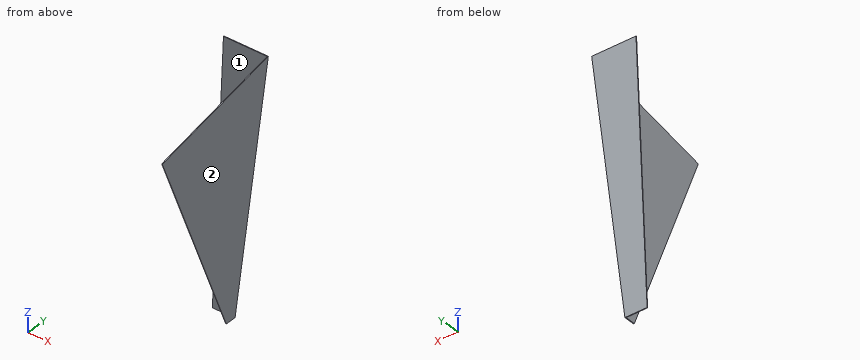
```python
from build123d import *

# Parameters (mm, degrees)
F1_DEPTH = 3.175
F3_DEPTH = 609.6
F5_DEPTH = 1211.58
F7_DEPTH = 25.4


with BuildPart() as f1:
    # F0 (on Front) → F1 (new body)
    with BuildSketch(Plane.XZ):
        Polygon((50.8, -609.6), (203.2, 609.6), (0, 609.6), (0, -609.6), align=None)
        Polygon((0, -609.6), (0, 609.6), (-203.2, 609.6), (-50.8, -609.6), align=None)
    extrude(amount=F1_DEPTH)

    # F2 (on face) → F3 (join)
    with BuildSketch(Plane.XZ.offset(3.175)):
        Polygon((47.6495177414, -609.2061897177), (50.8, -609.6), (203.2, 609.6), (200.0002914561, 609.6), align=None)
    extrude(amount=F3_DEPTH)

    # F4 (on face) → F5 (cut)
    with BuildSketch(Plane(origin=(125.0461538462, 0, -15.6307692308), x_dir=(0, 1, 0), z_dir=(0.9922778767, 0, -0.1240347346))):
        Polygon((-588.8283837058, 472.3203618187), (0, 630.0964517132), (0, 731.3741445541), (-712.4527692795, 731.3741445541), (-712.4527692795, -900.0895023346), (-50.8, -900.0895023346), (-50.8, -598.5916291275), align=None)
    extrude(amount=-F5_DEPTH, mode=Mode.SUBTRACT)

    # F6 (on face) → F7 (cut)
    with BuildSketch(Plane.XZ.offset(3.175)):
        Polygon((-203.2, 609.6), (-50.8, -609.6), (0, 609.6), align=None)
    extrude(amount=-F7_DEPTH, mode=Mode.SUBTRACT)


solid = f1.part
```
Verification items for the finished model (mm, model axes). Face numbers are marked on the shaded views. A direction names the side the tool comes from. Round coordinates to 2 decimals unless told otherwise and drop trailing zeros. Write each loop counter-clockwise with the first axis right and the second up, starting at its lowest first coordinate (ties: lowest second). Pieces come first, ordered by that corner, then holes. Notation, with made-up numbers: (58.5, 67) - (115.5, 67) arc R9 cw to (115.5, 74) - close; hole circle Ø5 at (-22, -30.75). An arc over 180 degrees is marked (long way). Answer as a JSON object with one key per item and string values. Group by question number.
Q1. Thickness scan on line 1 (Y direction, x = 149.5, z = 467) (3 decimals); line 2 (X direction, y = -394.5, z = 185.5); line 3 (X direction, y = -216, z = 151) (3 decimals). Record the ranges inside material, lowest first.
Q2. Section check B-B, the plane z = 160. Enter the section's corners in (x, y) (3 decimals), plus the area to 3 significant figures.
Q3. Section check C-C, the plane y = -522. Enter the section's corners in (x, z).
Q4. Section check D-D, the plane x = 107.5. Enter the section's corners in (y, z) (3 decimals), plus the area to 3 significant figures.
Q5. Go/stop test with flat-tipped pins: pin 1 Ø5 at (x, z) = (103, 131) entering from +Y; pin 2 Ø4 at (y, z) = (-304.5, 183) entering from +X (3 decimals); pin 3 Ø1.5 at (x, z) = (124.5, 183) entering from -Y (3 decimals); pin 4 Ø10 at (y, z) = (-96, 245) entering from -X. Record where each tip stops, or that it passes through.
Q6. Tool access check on the marked faces 1 and 2. Record the directions out of +Z, -Z, +X, -X, +Y, -Y that give a thin tool (end or side, any length) a straight path to the whole face; none if there is none.
Q7. Section check A-A, the plane x = 17. Enter the section's corners in (y, z) (3 decimals), plus the area to 3 significant figures.
Found:
{
 "1": {"line 1": "y = -3.175 to 0", "line 2": "x = 146.99 to 150.19", "line 3": "x = 142.675 to 145.875"},
 "2": {"outline": "(-18.733, -3.175) - (143.8, -3.175) - (143.8, -440.258) - (147, -440.458) - (147, 0) - (-18.733, 0) - close", "area": "1,930 mm^2"},
 "3": {"outline": "(163.98, 321.45) - (167.13, 321.05) - (185.85, 470.81) - (182.7, 471.2) - close"},
 "4": {"outline": "(-293.224, -130.402) - (-280.463, -156) - (0, -156) - (0, 609.6) - (-3.175, 609.6) - (-3.175, -130.402) - close", "area": "9,690 mm^2"},
 "5": {"pin 1": "stops at y = 0", "pin 2": "stops at x = 150.125", "pin 3": "stops at y = -3.175", "pin 4": "stops at x = 153.8"},
 "6": {"face 1": "+Z, -X, -Y", "face 2": "-Z, +X, +Y, -Y"},
 "7": {"outline": "(-3.175, -609.6) - (0, -609.6) - (0, 609.6) - (-3.175, 609.6) - close", "area": "3,870 mm^2"}
}
